```python
from build123d import *

# Parameters (mm, degrees)
SKETCH_1_W          = 160
SKETCH_1_H          = 105
EXTRUDE_1_DEPTH     = 5
SKETCH_2_R          = 1.7
CUT_EXTRUDE_1_DEPTH = 200
SKETCH_3_R          = 1.7
CUT_EXTRUDE_2_DEPTH = 200


with BuildPart() as part:
    # 草图1 → 凸台-拉伸1 (new body)
    with BuildSketch(Plane(origin=(0, 0, 0), x_dir=(1, 0, 0), z_dir=(0, 1, 0))):
        Rectangle(SKETCH_1_W, SKETCH_1_H)
    extrude(amount=EXTRUDE_1_DEPTH)

    # 草图2 → 切除-拉伸1 (cut)
    with BuildSketch(Plane(origin=(80, 0, 0), x_dir=(0, 0, -1), z_dir=(1, 0, 0))):
        with Locations((-2.5, 2.5)):
            Circle(SKETCH_2_R)
    extrude(amount=-CUT_EXTRUDE_1_DEPTH, mode=Mode.SUBTRACT)

    # 草图3 → 切除-拉伸2 (cut)
    with BuildSketch(Plane(origin=(80, 0, 0), x_dir=(0, 0, -1), z_dir=(1, 0, 0))):
        with Locations((50, 2.5)):
            Circle(SKETCH_3_R)
    extrude(amount=-CUT_EXTRUDE_2_DEPTH, mode=Mode.SUBTRACT)


solid = part.part
```
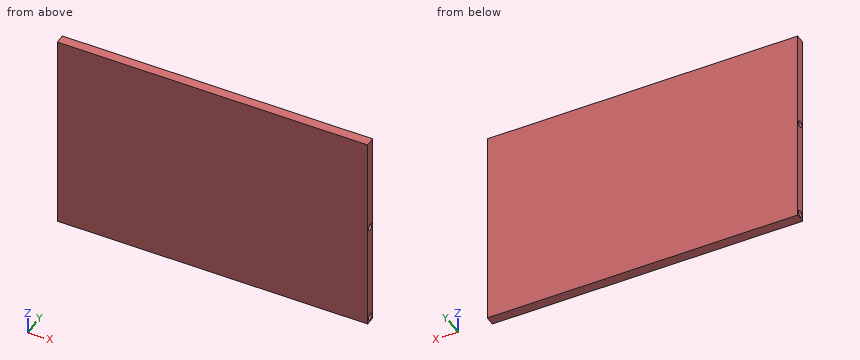
Model file for the job. Use its own axes, mm. Coordinates: 2 decimals unless noted, no trailing zeros. Order: outer loops, then holes, each group sorted by start corner. A loop starts at its lowest first (then second) coordinate and runs counter-clockwise, first axis right, second up. Notation, with made-up numbers: (9.5, -10.75) -> (47.5, -10.75) arc R22 ccw to (47.5, 6.25) -> close; hole circle Ø3 at (68, 24.25). An arc over 180 degrees is marked (long way). Answer as a JSON object with one key per item and string values. Group by question number.
1) Drill centre lines: L1, parallel to Z at x = -60, y = 2.75; L2, parallel to Z at x = 24, y = 3.9; L3, parallel to Y at x = 45.5, z = 2.5. Where is each one in solid material? Low to high.
2) Cut at A-A, the plane z = -50. Write the cut outline in (x, y), then the cut area to 3 significant figures.
3) Cut at B-B, the plane x = -21. Write the cut outline in (y, z), then the cut area to 3 significant figures.
Check values:
{
 "1": {"L1": "z = -52.5 to -51.68, -48.32 to 0.82, 4.18 to 52.5", "L2": "z = -52.5 to -50.96, -49.04 to 1.54, 3.46 to 52.5", "L3": "y = 0 to 0.8, 4.2 to 5"},
 "2": {"outline": "(-80, 0) -> (80, 0) -> (80, 0.8) -> (-80, 0.8) -> close; (-80, 4.2) -> (80, 4.2) -> (80, 5) -> (-80, 5) -> close", "area": "256 mm²"},
 "3": {"outline": "(0, -52.5) -> (5, -52.5) -> (5, 52.5) -> (0, 52.5) -> close; hole circle Ø3.4 at (2.5, -50); hole circle Ø3.4 at (2.5, 2.5)", "area": "507 mm²"}
}
